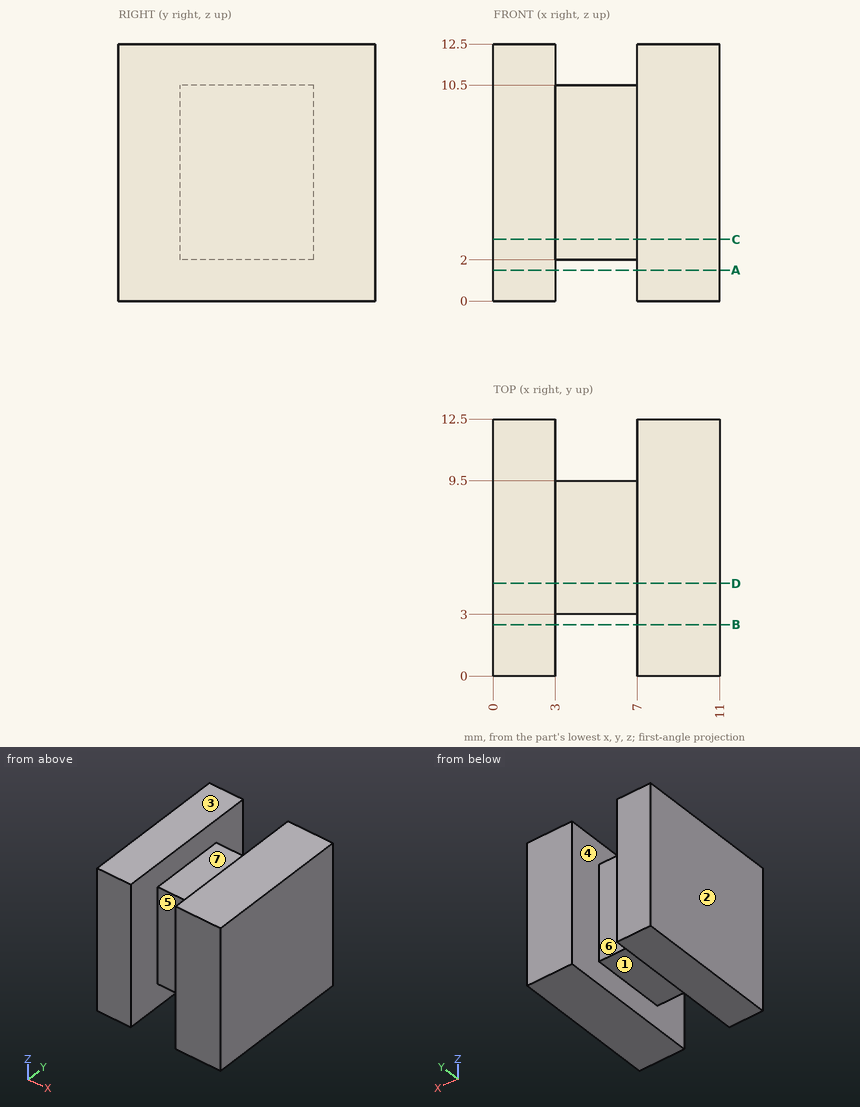
Verification items for this drawing (mm, ordinates from the low corner). A direction names the side the tool comes from. Round coordinates to 2 decimals unless told otherwise and drop trailing zeros. Order: outer loops, then holes, each group sorted by start corner. A loop starts at its lowest first (then second) coordinate and runs counter-clockwise, first axis right, second up. Notation, with made-up numbers: M -5,-10 L 45,-10 A20 cw 45,2 Z; hole C 20.5,-5.5 d9. An arc over 180 degrees is marked long. Answer in a Markdown table with one row per item. Add a question column.
Item 1: Material ranges on L1, parallel to X at y = 7.25, z = 10.75; L2, parallel to Z at x = 4.5, y = 9; L3, parallel to Y at x = 4.25, z = 4.5, recorded low to high. Write a range as [from, to].
Item 2: Draft check along X on the marked faces 1, 2, 3 and 4. Enter one of: released by +X, released by -X, zero draft, split by the parting line, or undercut.
Item 3: Depth check by flat-ended pin: pin 1 Ø1.5 at (x, z) = (7, 8) entering from -Y; pin 2 Ø2 at (x, y) = (5, 5.5) entering from -Z; pin 3 Ø1.2 at (x, z) = (5, 5) entering from +Y; pin 4 Ø2 at (x, z) = (5.5, 4.5) entering from -Y. Enter the tip coordinate at first touch or a pass-through.
Item 4: Sectioned sample at A-A, the plane z = 1.5. Enter the section's corners in (x, y).
Item 5: Set-up check for the marked faces 5, 6 and 7: record each of +Z, -Z, +X, -X, +Y, -Y from which the full face is reachable in a straight line by a thin tool's end or side.
Item 6: Sectioned sample at D-D, the plane y = 4.5. Enter the section's corners in (x, z).
Item 7: Sectioned sample at C-C, the plane z = 3. Enter the section's corners in (x, y).
Filled in:
| question | item | result |
|---|---|---|
| 1 | L1 | x = [0, 3], [7, 11] |
| 1 | L2 | z = [2, 10.5] |
| 1 | L3 | y = [3, 9.5] |
| 2 | face 1 | undercut |
| 2 | face 2 | released by -X |
| 2 | face 3 | zero draft |
| 2 | face 4 | undercut |
| 3 | pin 1 | stops at y = 0 |
| 3 | pin 2 | stops at z = 2 |
| 3 | pin 3 | stops at y = 9.5 |
| 3 | pin 4 | stops at y = 3 |
| 4 | outline | M 0,0 L 3,0 L 3,12.5 L 0,12.5 Z; M 7,0 L 11,0 L 11,12.5 L 7,12.5 Z |
| 5 | face 5 | +Z, -Z, -Y |
| 5 | face 6 | +Z, -Z, +Y |
| 5 | face 7 | +Z, +Y, -Y |
| 6 | outline | M 0,0 L 3,0 L 3,2 L 7,2 L 7,0 L 11,0 L 11,12.5 L 7,12.5 L 7,10.5 L 3,10.5 L 3,12.5 L 0,12.5 Z |
| 7 | outline | M 0,0 L 3,0 L 3,3 L 7,3 L 7,0 L 11,0 L 11,12.5 L 7,12.5 L 7,9.5 L 3,9.5 L 3,12.5 L 0,12.5 Z |
